Build history of the part. All positions in model axes, mm. A direction names the side the tool comes from. Round coordinates to 2 decimals unless told otherwise and drop trailing zeros. Order: outer loops, then holes, each group sorted by start corner. A loop starts at its lowest first (then second) coordinate and runs counter-clockwise, first axis right, second up. Notation, with made-up numbers: (-38, -21) -> (-17, -21) arc R14 cw to (-17, -17) -> close; hole circle Ø3 at (9.5, 30). An arc over 180 degrees is marked (long way). Use a Markdown table: item, result. Add a question column.
Item 1: Slice it at D-D, the plane z = -21. Give the cut face in (x, y).
Item 2: Pin check, flat tips, straight feed: pin 1 (0.6 mm diameter, centred on x = 62.5, z = -27.5, fed in from +Y); pin 2 (1.4 mm diameter, centred on x = -62.5, z = -26, fed in from -Y); pin 3 (0.5 mm diameter, centred on x = -50, y = -177, fed in from +Z). Stop position of each tip, or through.
Item 3: Slice it at C-C, the plane y = -95. Give the cut face in (x, z).
Item 4: Slice it at A-A, the plane x = -50.5. Give the cut face in (y, z).
Item 5: 3-axis set-ups, long thin cutter, end or side, ignore diameter. For faces 1 (the face through (-5, -78, 0)), 2 (the face through (-1, -128, -39)): which of +Z, -Z, +X, -X, +Y, -Y reach the whole face in a straight line?
Item 6: Slice it at B-B, the plane z = -12. Give the cut face in (x, y).
Item 7: Probe L1, parallel to X at y = -125, z = -17.5; L2, parallel to Y at x = -2, z = -26; L3, parallel to X at y = -71, z = -11. List the from-to ranges inside material, lowest first.
Item 8: Two-plate mould, pull along X, no slides. Class faces 3 (the face through (63.158, -113, -20)), 4 (the face through (-1, -127, -40)), 5 (the face through (-18.91, -176.96, -3.18)): released by +X, released by -X, zero draft, split by the parting line, or undercut.
from build123d import *

# Parameters (mm, degrees)
BOSS_EXTRUDE1_DEPTH     = 40
SKETCH3_W               = 1.255387907
SKETCH3_H               = 40
BOSS_EXTRUDE2_DEPTH     = 130
SKETCH4_W               = 126.316334496
SKETCH4_H               = 1
BOSS_EXTRUDE3_DEPTH     = 150
SKETCH5_R               = 78
CUT_EXTRUDE3_DEPTH      = 90
SKETCH6_W               = 126.316334496
SKETCH6_H               = 1
BOSS_EXTRUDE4_DEPTH     = 39
CUT_EXTRUDE4_DEPTH      = 39
CUT_EXTRUDE5_DEPTH      = 152.425375183
CUT_EXTRUDE5_DEPTH_BACK = 1
SKETCH8_W               = 20
SKETCH8_H               = 5
SKETCH8_H_2             = 28
SKETCH9_R               = 15.335640517
CUT_EXTRUDE6_DEPTH      = 1


with BuildPart() as part:
    # Sketch2 → Boss-Extrude1 (new body)
    with BuildSketch(Plane.XY):
        with BuildLine():
            Line((61.902779341, -47.455725786), (63.158167248, -47.455725786))
            ThreePointArc((63.158167248, -47.455725786), (0, -79), (-63.158167248, -47.455725786))
            Line((-63.158167248, -47.455725786), (-61.902779341, -47.455725786))
            ThreePointArc((-61.902779341, -47.455725786), (0, -78), (61.902779341, -47.455725786))
        make_face()
    extrude(amount=-BOSS_EXTRUDE1_DEPTH)

    # Sketch3 → Boss-Extrude2 (add)
    with BuildSketch(Plane(origin=(0, -47.455725786, 0), x_dir=(1, 0, 0), z_dir=(0, 1, 0))):
        with Locations((-62.530473295, 20)):
            Rectangle(SKETCH3_W, SKETCH3_H)
        with Locations((62.530473295, 20)):
            Rectangle(SKETCH3_W, SKETCH3_H)
    extrude(amount=-BOSS_EXTRUDE2_DEPTH)

    # Sketch4 → Boss-Extrude3 (add)
    with BuildSketch(Plane.XZ.offset(177.455725786)):
        with Locations((0, -39.5)):
            Rectangle(SKETCH4_W, SKETCH4_H)
    extrude(amount=-BOSS_EXTRUDE3_DEPTH)

    # Sketch5 → Cut-Extrude3 (cut)
    with BuildSketch(Plane.XY.offset(-39)):
        Circle(SKETCH5_R)
    extrude(amount=-CUT_EXTRUDE3_DEPTH, mode=Mode.SUBTRACT)

    # Sketch6 → Boss-Extrude4 (add)
    with BuildSketch(Plane.XY.offset(-39)):
        with Locations((0, -176.955725786)):
            Rectangle(SKETCH6_W, SKETCH6_H)
    extrude(amount=BOSS_EXTRUDE4_DEPTH)

    # Sketch7 → Cut-Extrude4 (cut)
    with BuildSketch(Plane.XZ.offset(177.455725786)):
        with BuildLine():
            Line((0, 0), (-30, 0))
            ThreePointArc((-30, 0), (0, -2.075596442), (30, 0))
            Line((30, 0), (0, 0))
        make_face()
    extrude(amount=-CUT_EXTRUDE4_DEPTH, mode=Mode.SUBTRACT)

    # Sketch8 → Cut-Extrude5 (cut, two sides: drawn at the far end of the back side and taken through both)
    with BuildSketch(Plane.XZ.offset(177.455725786).offset(-CUT_EXTRUDE5_DEPTH_BACK)):
        with Locations((-51.658167248, -2.5)):
            Rectangle(SKETCH8_W, SKETCH8_H)
        with Locations((-53.158167248, -21)):
            Rectangle(SKETCH8_W, SKETCH8_H_2)
    extrude(amount=CUT_EXTRUDE5_DEPTH + CUT_EXTRUDE5_DEPTH_BACK, mode=Mode.SUBTRACT)

    # Sketch9 → Cut-Extrude6 (cut)
    with BuildSketch(Plane.XZ.offset(177.455725786)):
        with Locations(Location((-19.587676617, -18.499331227, 0), (0, 0, 270))):
            Circle(SKETCH9_R)
    extrude(amount=-CUT_EXTRUDE6_DEPTH, mode=Mode.SUBTRACT)


solid = part.part
Check sheet entries:
| question | item | result |
|---|---|---|
| 1 | outline | (-63.16, -176.46) -> (-61.9, -176.46) -> (-61.9, -49.08) arc R79 ccw to (61.9, -49.08) -> (61.9, -176.46) -> (-4.46, -176.46) -> (-4.46, -177.46) -> (63.16, -177.46) -> (63.16, -47.46) -> (61.9, -47.46) arc R78 cw to (-61.9, -47.46) -> (-63.16, -47.46) -> close; (-43.16, -177.46) -> (-34.72, -177.46) -> (-34.72, -176.46) -> (-43.16, -176.46) -> close |
| 2 | pin 1 | y = -47.46 |
| 2 | pin 2 | y = -176.46 |
| 2 | pin 3 | z = -5 |
| 3 | outline | (-63.16, -40) -> (63.16, -40) -> (63.16, 0) -> (61.9, 0) -> (61.9, -39) -> (-61.9, -39) -> (-61.9, 0) -> (-63.16, 0) -> close |
| 4 | outline | (-177.46, -40) -> (-59.45, -40) -> (-59.45, 0) -> (-60.75, 0) -> (-60.75, -39) -> (-176.46, -39) -> (-176.46, -35) -> (-177.46, -35) -> close; (-177.46, -7) -> (-176.46, -7) -> (-176.46, -5) -> (-177.46, -5) -> close |
| 5 | face 1 | +Z, +X, -X, +Y, -Y |
| 5 | face 2 | +Z |
| 6 | outline | (-63.16, -176.46) -> (-61.9, -176.46) -> (-61.9, -49.08) arc R79 ccw to (61.9, -49.08) -> (61.9, -176.46) -> (-5.7, -176.46) -> (-5.7, -177.46) -> (63.16, -177.46) -> (63.16, -47.46) -> (61.9, -47.46) arc R78 cw to (-61.9, -47.46) -> (-63.16, -47.46) -> close; (-43.16, -177.46) -> (-33.48, -177.46) -> (-33.48, -176.46) -> (-43.16, -176.46) -> close |
| 7 | L1 | -63.16 to -61.9, 61.9 to 63.16 |
| 7 | L2 | -177.46 to -176.46, -78.97 to -77.97 |
| 7 | L3 | -63.16 to -61.9, -34.64 to -32.3, 32.3 to 34.64, 61.9 to 63.16 |
| 8 | face 3 | released by +X |
| 8 | face 4 | zero draft |
| 8 | face 5 | undercut |
